Source: CAD feature listing. Evaluate the final solid. Frame: model axes, mm. A direction names the side the tool comes from. Give positions to 0.01 mm unless a question says otherwise; leave off trailing zeros. Write each loop counter-clockwise with the first axis right and the second up, starting at its lowest first coordinate (ties: lowest second). Pieces come first, ordered by that corner, then holes. Notation, with made-up numbers: (-6, 31) -> (42, 31) arc R22 cw to (42, 43) -> close; hole circle Ø7 at (73.25, 19.5). An arc over 180 degrees is marked (long way). Use one line per item in the form item = value. Start each with the question number.
(1) Material intervals for line 1 along Z through (x, y) = (6, -36); line 2 along Z through (x, y) = (0.5, -10); line 3 along Z through (x, y) = (6.5, -34.5), sorted ascending. Write a range as from..to.
(2) Cut plane B-B, the plane x = -13. Output: boundary loops of the cut face in (y, z), and give its area (3 significant figures).
(3) First-contact query: P1, Ø1.5, axis at x = 22, y = 20, coming from the -Z side; P2, Ø1.5, axis at y = -8, z = -13, coming from the +X side; P3, Ø8, axis at x = 8.5, y = 3.5, coming from the -Z side. Flat tips, straight axial feed; report the tip coordinate or a pass-through.
(4) Set-up query: faces 1 (the face through (-11.4, -35.2, -1.2)), 2 (the face through (-0.2, -33, -10.4)), 3 (the face through (-9, 0, -40)). Return all of +Z, -Z, +X, -X, +Y, -Y with unobstructed straight access to the full face (end or side cutting, diameter ignored); none if empty.
(5) Draft query along X for faces 4 (the face through (7.974, -35.218, -9.907)), 5 (the face through (-1, 30, 1)), 6 (the face through (-2.17, -31.48, -9.76)). Return one class per face: pulls with the +X half, pulls with the -X half, needs draft (parallel to the pull), parting line crosses it, or undercut.
(6) Cut plane D-D, the plane y = -18. Output: boundary loops of the cut face in (x, z), and give its area (3 significant figures).
(7) Cut plane A-A, the plane z = 0. Output: boundary loops of the cut face in (x, y), and give its area (3 significant figures).
(8) Cut plane C-C, the plane x = 0. Output: boundary loops of the cut face in (y, z), and give its area (3 significant figures).
from build123d import *

# Parameters (mm, degrees)
F0_R            = 41
F1_DEPTH        = 30
F1_DEPTH_BACK   = 30
F2_R            = 10
F3_DEPTH        = 3
F4_R            = 16
F5_DEPTH        = 4.5
F7_D            = 4
F7_DEPTH        = 5
F7_TIP          = 1.2017212381
F7_COPIES_COUNT = 3


# Not quite as in the source:
# - a pattern or mirror of a feature is missing from the dataset's text; its kind, count and spacing are read off the source's solid


with BuildPart() as f1:
    # F0 (on Front) → F1 (new body, two sides)
    with BuildSketch(Plane.XZ) as f1_sk:
        Circle(F0_R)
    extrude(amount=F1_DEPTH)
    extrude(f1_sk.sketch, amount=-F1_DEPTH_BACK)

    # F2 (on face) → F3 (join)
    with BuildSketch(Plane.XZ.offset(30)):
        Circle(F2_R)
    extrude(amount=F3_DEPTH)

    # F4 (on face) → F5 (join)
    with BuildSketch(Plane.XZ.offset(33)):
        Circle(F4_R)
    extrude(amount=F5_DEPTH)

    # F7
    with Locations(Plane.XZ.offset(37.5)):
        with Locations((-13, 0)):
            f7 = Hole(F7_D / 2, depth=F7_DEPTH)
            with Locations((0, 0, -(F7_DEPTH + F7_TIP / 2))):  # 118° drill point
                Cone(0, F7_D / 2, F7_TIP, mode=Mode.SUBTRACT)

    # F7_copies: F7 ×3 about axis
    f7_copies_axis = Axis((0, 0, 0), (0, 1, 0))
    for i in range(1, F7_COPIES_COUNT):
        add(f7.rotate(f7_copies_axis, i * 360 / F7_COPIES_COUNT), mode=Mode.SUBTRACT)


solid = f1.part
Geometry says:
q1.line_1 = -14.83..-13.19, -9.32..9.32, 13.19..14.83
q1.line_2 = -41..41
q1.line_3 = -14.62..-13.26, -9.26..9.26, 13.26..14.62
q2.outline = (-37.5, -9.33) -> (-33, -9.33) -> (-33, -2) -> (-37.5, -2) -> close; (-37.5, 2) -> (-33, 2) -> (-33, 9.33) -> (-37.5, 9.33) -> close; (-30, -38.88) -> (30, -38.88) -> (30, 38.88) -> (-30, 38.88) -> close
q2.area = 4,730 mm^2
q3.P1 = -35.06
q3.P2 = 39.13
q3.P3 = -40.75
q4.face_1 = -Y
q4.face_2 = none
q4.face_3 = +Y, -Y
q5.face_4 = undercut
q5.face_5 = needs draft
q5.face_6 = parting line crosses it
q6.outline = circle Ø82 at (0, 0)
q6.area = 5,280 mm^2
q7.outline = (-41, -30) -> (-10, -30) -> (-10, -33) -> (-11, -33) -> (-11, -37.5) -> (16, -37.5) -> (16, -33) -> (10, -33) -> (10, -30) -> (41, -30) -> (41, 30) -> (-41, 30) -> close; (-16, -37.5) -> (-15, -37.5) -> (-15, -33) -> (-16, -33) -> close
q7.area = 5,110 mm^2
q8.outline = (-37.5, -16) -> (-33, -16) -> (-33, -10) -> (-30, -10) -> (-30, -41) -> (30, -41) -> (30, 41) -> (-30, 41) -> (-30, 10) -> (-33, 10) -> (-33, 16) -> (-37.5, 16) -> close
q8.area = 5,120 mm^2
